```python
from build123d import *

# Parameters (mm, degrees)
SKETCH_8_R      = 2
SKETCH_8_R_2    = 5
SKETCH_8_R_3    = 1.5
EXTRUDE_1_DEPTH = 1.6


with BuildPart() as part:
    # 草图8 → 凸台-拉伸1 (new body)
    with BuildSketch(Plane.XZ):
        with BuildLine():
            Line((30.529437252, 84), (36.227922061, 89.69848481))
            ThreePointArc((36.227922061, 89.69848481), (36.935028843, 89.991378029), (37.642135624, 89.69848481))
            Line((37.642135624, 89.69848481), (53.19848481, 74.142135624))
            ThreePointArc((53.19848481, 74.142135624), (53.491378029, 73.435028843), (53.19848481, 72.727922061))
            Line((53.19848481, 72.727922061), (47.5, 67.029437252))
            ThreePointArc((47.5, 67.029437252), (42.297453968, 59.24327688), (40.470562748, 50.058874503))
            Line((40.470562748, 50.058874503), (40.470562748, 36))
            ThreePointArc((40.470562748, 36), (47.5, 19.029437252), (64.470562748, 12))
            Line((64.470562748, 12), (77.470562748, 12))
            ThreePointArc((77.470562748, 12), (78.17766953, 11.707106781), (78.470562748, 11))
            Line((78.470562748, 11), (78.470562748, -11))
            ThreePointArc((78.470562748, -11), (78.17766953, -11.707106781), (77.470562748, -12))
            Line((77.470562748, -12), (64.470562748, -12))
            ThreePointArc((64.470562748, -12), (47.5, -19.029437252), (40.470562748, -36))
            Line((40.470562748, -36), (40.470562748, -50.058874503))
            ThreePointArc((40.470562748, -50.058874503), (42.297453968, -59.24327688), (47.5, -67.029437252))
            Line((47.5, -67.029437252), (53.19848481, -72.727922061))
            ThreePointArc((53.19848481, -72.727922061), (53.491378029, -73.435028843), (53.19848481, -74.142135624))
            Line((53.19848481, -74.142135624), (37.642135624, -89.69848481))
            ThreePointArc((37.642135624, -89.69848481), (36.935028843, -89.991378029), (36.227922061, -89.69848481))
            Line((36.227922061, -89.69848481), (30.529437252, -84))
            ThreePointArc((30.529437252, -84), (22.74327688, -78.797453968), (13.558874503, -76.970562748))
            Line((13.558874503, -76.970562748), (-13.558874503, -76.970562748))
            ThreePointArc((-13.558874503, -76.970562748), (-22.74327688, -78.797453968), (-30.529437252, -84))
            Line((-30.529437252, -84), (-36.227922061, -89.69848481))
            ThreePointArc((-36.227922061, -89.69848481), (-36.935028843, -89.991378029), (-37.642135624, -89.69848481))
            Line((-37.642135624, -89.69848481), (-53.19848481, -74.142135624))
            ThreePointArc((-53.19848481, -74.142135624), (-53.491378029, -73.435028843), (-53.19848481, -72.727922061))
            Line((-53.19848481, -72.727922061), (-47.5, -67.029437252))
            ThreePointArc((-47.5, -67.029437252), (-42.297453968, -59.24327688), (-40.470562748, -50.058874503))
            Line((-40.470562748, -50.058874503), (-40.470562748, -36))
            ThreePointArc((-40.470562748, -36), (-47.5, -19.029437252), (-64.470562748, -12))
            Line((-64.470562748, -12), (-77.470562748, -12))
            ThreePointArc((-77.470562748, -12), (-78.17766953, -11.707106781), (-78.470562748, -11))
            Line((-78.470562748, -11), (-78.470562748, 11))
            ThreePointArc((-78.470562748, 11), (-78.17766953, 11.707106781), (-77.470562748, 12))
            Line((-77.470562748, 12), (-64.470562748, 12))
            ThreePointArc((-64.470562748, 12), (-47.5, 19.029437252), (-40.470562748, 36))
            Line((-40.470562748, 36), (-40.470562748, 50.058874503))
            ThreePointArc((-40.470562748, 50.058874503), (-42.297453968, 59.24327688), (-47.5, 67.029437252))
            Line((-47.5, 67.029437252), (-53.19848481, 72.727922061))
            ThreePointArc((-53.19848481, 72.727922061), (-53.491378029, 73.435028843), (-53.19848481, 74.142135624))
            Line((-53.19848481, 74.142135624), (-37.642135624, 89.69848481))
            ThreePointArc((-37.642135624, 89.69848481), (-36.935028843, 89.991378029), (-36.227922061, 89.69848481))
            Line((-36.227922061, 89.69848481), (-30.529437252, 84))
            ThreePointArc((-30.529437252, 84), (-22.74327688, 78.797453968), (-13.558874503, 76.970562748))
            Line((-13.558874503, 76.970562748), (13.558874503, 76.970562748))
            ThreePointArc((13.558874503, 76.970562748), (22.74327688, 78.797453968), (30.529437252, 84))
        make_face()
        with Locations(Location((-39.056349186, 64.242640687, 0), (0, 0, 90))):
            Circle(SKETCH_8_R, mode=Mode.SUBTRACT)
        with Locations(Location((-27.742640687, 75.556349186, 0), (0, 0, 90))):
            Circle(SKETCH_8_R, mode=Mode.SUBTRACT)
        with Locations(Location((0, 26.970562748, 0), (0, 0, 90))):
            Circle(SKETCH_8_R_2, mode=Mode.SUBTRACT)
        with Locations(Location((-61.470562748, 8, 0), (0, 0, 90))):
            Circle(SKETCH_8_R, mode=Mode.SUBTRACT)
        with Locations(Location((-25.887975085, -10.446849588, 0), (0, 0, 90))):
            Circle(SKETCH_8_R_3, mode=Mode.SUBTRACT)
        with Locations(Location((-25.887975085, 64.387975085, 0), (0, 0, 90))):
            Circle(SKETCH_8_R_3, mode=Mode.SUBTRACT)
        with Locations(Location((27.742640687, -75.556349186, 0), (0, 0, 90))):
            Circle(SKETCH_8_R, mode=Mode.SUBTRACT)
        with Locations(Location((39.056349186, -64.242640687, 0), (0, 0, 90))):
            Circle(SKETCH_8_R, mode=Mode.SUBTRACT)
        with Locations(Location((-27.742640687, -75.556349186, 0), (0, 0, 90))):
            Circle(SKETCH_8_R, mode=Mode.SUBTRACT)
        with Locations(Location((-39.056349186, -64.242640687, 0), (0, 0, 90))):
            Circle(SKETCH_8_R, mode=Mode.SUBTRACT)
        with Locations(Location((13.427835179, -71.170562748, 0), (0, 0, 90))):
            Circle(SKETCH_8_R_3, mode=Mode.SUBTRACT)
        with Locations(Location((-13.1297961, -71.170562748, 0), (0, 0, 90))):
            Circle(SKETCH_8_R_3, mode=Mode.SUBTRACT)
        with Locations(Location((-61.470562748, -8, 0), (0, 0, 90))):
            Circle(SKETCH_8_R, mode=Mode.SUBTRACT)
    extrude(amount=EXTRUDE_1_DEPTH)


solid = part.part
```
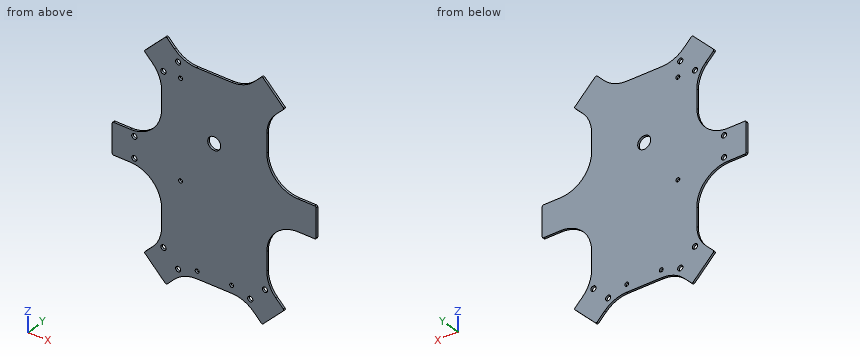
Geometry check sheet. Reference: the model listing, model coordinates, mm. Coordinates: 2 decimals unless noted, no trailing zeros. Loops run counter-clockwise (first coordinate to the right, second up) from the corner with the lowest first, then second, coordinate; pieces in that order, holes last. Notation, with made-up numbers: (55.25, 54) - (109.25, 54) arc R28 cw to (109.25, 76) - close; hole circle Ø8 at (72.5, 34.5). An arc over 180 degrees is marked (long way). One line per item, written item: value. Start each with the question number.
(1) Cross-section at A-A on z = 8. Enter the section's corners in (x, y).
(2) Cross-section at D-D on y = -1. Count the separate pieces of the cut face and the enclosed holes in it, plus the area to 3 significant figures.
(3) Cross-section at B-B on x = 0. Enter the section's corners in (y, z), plus the area to 3 significant figures.
(4) Cross-section at C-C on x = -44. Enter the section's corners in (y, z).
(5) Material ranges on line 1 (Z direction, x = 53, y = -1); line 2 (X direction, y = -0.5, z = -8); line 3 (X direction, y = -1.05, z = 49.5), recorded low to high. Write a range as [from, to].
(6) Depth check by flat-ended pin: P1, Ø0.8, axis at x = 72.5, y = -0.5, coming from the +Z side; P2, Ø0.8, axis at x = -70.5, y = -1, coming from the -Z side; P3, Ø6.5, axis at x = -27.74, z = 75.56, coming from the +Y side. Enter the tip coordinate at first touch or a pass-through.
Results below:
1. outline: (-78.47, -1.6) - (-63.47, -1.6) - (-63.47, 0) - (-78.47, 0) - close; (-59.47, -1.6) - (78.47, -1.6) - (78.47, 0) - (-59.47, 0) - close
2. separate pieces: 1
2. enclosed holes: 13
2. area: 15,900 mm2
3. outline: (-1.6, -76.97) - (0, -76.97) - (0, 21.97) - (-1.6, 21.97) - close; (-1.6, 31.97) - (0, 31.97) - (0, 76.97) - (-1.6, 76.97) - close
3. area: 230 mm2
4. outline: (-1.6, -83.34) - (0, -83.34) - (0, -62.59) - (-1.6, -62.59) - close; (-1.6, -23.47) - (0, -23.47) - (0, 23.47) - (-1.6, 23.47) - close; (-1.6, 62.59) - (0, 62.59) - (0, 83.34) - (-1.6, 83.34) - close
5. line 1: z = [-74.34, -72.53], [-14.92, 14.92], [72.53, 74.34]
5. line 2: x = [-78.47, -63.47], [-59.47, 78.47]
5. line 3: x = [-40.47, 40.47]
6. P1: stops at z = 12
6. P2: stops at z = -12
6. P3: stops at y = 0
